Part model, mm, in its own coordinate system. A direction names the side the tool comes from. Give positions to 0.01 mm unless a question says otherwise; leave off trailing zeros. Order: outer loops, then holes, each group sorted by start corner. A loop starts at its lowest first (then second) coordinate and runs counter-clockwise, first axis right, second up. Notation, with made-up numbers: M 2,-29.5 L 16,-29.5 A20 ccw 16,3.5 Z; hole C -26,17 d9. An arc over 180 degrees is marked long. Return JSON: item names as keys, results as strings.
Autodesk Inventor part; units mm, degrees
ref_plane "YZ Plane" through (0, 0, 0) normal (1, 0, 0) x (0, 1, 0)
ref_plane "XZ Plane" through (0, 0, 0) normal (0, 1, 0) x (-1, 0, 0)
ref_plane "XY Plane" through (0, 0, 0) normal (0, 0, 1) x (1, 0, 0)
sketch "Boceto1" plane through (0, 0, 0) normal (0, 0, 1) x (1, 0, 0)
  line L0 (0, 0) -> (177, 0)
  line L1 (177, 0) -> (177, 127.5)
  line L2 (177, 127.5) -> (0, 127.5)
  line L3 (0, 127.5) -> (0, 0)
  line L4 (0, 127.5) -> (11.5, 127.5)
  line L5 (11.5, 127.5) -> (11.5, 116)
  line L6 (11.5, 116) -> (0, 116)
  line L7 (0, 116) -> (0, 127.5)
  line L8 (177, 0) -> (165.5, 0)
  line L9 (165.5, 0) -> (165.5, 11.5)
  line L10 (165.5, 11.5) -> (177, 11.5)
  line L11 (177, 11.5) -> (177, 0)
  line L12 (11.5, 116) -> (165.5, 116)
  line L13 (165.5, 116) -> (165.5, 11.5)
  line L14 (165.5, 11.5) -> (11.5, 11.5)
  line L15 (11.5, 11.5) -> (11.5, 116)
  dimension "d0" = 177
  dimension "d1" = 127.5
  dimension "d2" = 11.5
  dimension "d3" = 11.5
  dimension "d4" = 11.5
  dimension "d5" = 11.5
extrude "Extrusión1" add sketch "Boceto1" along normal blind 30 contours L3 L6 L15 L14 L9 L0 | L9 L10 L1 L0 | L3 L2 L5 L6 | L13 L12 L5 L2 L1 L10
sketch "Boceto2" plane through (0, 0, 30) normal (0, 0, 1) x (1, 0, 0)
  line L0 (11.5, 116) -> (6.5, 116)
  line L1 (6.5, 116) -> (6.5, 11.5)
  line L2 (6.5, 11.5) -> (11.5, 11.5)
  line L3 (11.5, 11.5) -> (11.5, 116)
  line L4 (165.5, 116) -> (170.5, 116)
  line L5 (170.5, 116) -> (170.5, 11.5)
  line L6 (170.5, 11.5) -> (165.5, 11.5)
  line L7 (165.5, 11.5) -> (165.5, 116)
  line L8 (11.5, 116) -> (165.5, 116)
  line L9 (165.5, 116) -> (165.5, 119.75)
  line L10 (165.5, 119.75) -> (11.5, 119.75)
  line L11 (11.5, 119.75) -> (11.5, 116)
  line L12 (11.5, 11.5) -> (165.5, 11.5)
  line L13 (165.5, 11.5) -> (165.5, 7.75)
  line L14 (165.5, 7.75) -> (11.5, 7.75)
  line L15 (11.5, 7.75) -> (11.5, 11.5)
  dimension "d30" = 5
  dimension "d31" = 5
  dimension "d32" = 104.5
  dimension "d33" = 3.75
  dimension "d34" = 3.75
extrude "Extrusión2" cut sketch "Boceto2" against normal blind 30 contours L3 L2 L1 L0 | L11 L10 L9 L8 | L12 L13 L14 L15 | L4 L5 L6 L7
sketch "Boceto3" plane through (0, 0, 30) normal (0, 0, 1) x (1, 0, 0)
  line L0 (177, 0) -> (171.25, 0)
  line L1 (171.25, 0) -> (171.25, 5.75)
  line L2 (171.25, 5.75) -> (177, 5.75)
  line L3 (177, 5.75) -> (177, 0)
  line L4 (0, 0) -> (5.75, 0)
  line L5 (5.75, 0) -> (5.75, 5.75)
  line L6 (5.75, 5.75) -> (0, 5.75)
  line L7 (0, 5.75) -> (0, 0)
  line L8 (0, 127.5) -> (5.75, 127.5)
  line L9 (5.75, 127.5) -> (5.75, 121.75)
  line L10 (5.75, 121.75) -> (0, 121.75)
  line L11 (0, 121.75) -> (0, 127.5)
  line L12 (177, 127.5) -> (171.25, 127.5)
  line L13 (171.25, 127.5) -> (171.25, 121.75)
  line L14 (171.25, 121.75) -> (177, 121.75)
  line L15 (177, 121.75) -> (177, 127.5)
  circle A0 centre (5.75, 121.75) radius 2
  circle A1 centre (171.25, 121.75) radius 2
  circle A2 centre (171.25, 5.75) radius 2
  circle A3 centre (5.75, 5.75) radius 2
  dimension "d16" = 5.75
  dimension "d17" = 5.75
  dimension "d18" = 5.75
  dimension "d19" = 5.75
  dimension "d20" = 5.75
  dimension "d21" = 5.75
  dimension "d22" = 5.75
  dimension "d23" = 5.75
  dimension "d24" = 4
  dimension "d25" = 4
  dimension "d26" = 4
  dimension "d27" = 4
extrude "Extrusión3" cut sketch "Boceto3" against normal blind 30 contours A2 L2 L1 | L1 L2 A2 | A3 L6 L5 | L5 L6 A3 | A0 L10 L9 | L9 L10 A0 | A1 L14 L13 | L13 L14 A1
sketch "Boceto4" plane through (0, 0, 0) normal (0, -1, 0) x (1, 0, 0)
  line L0 (0, 30) -> (21.5, 30)
  line L1 (21.5, 30) -> (21.5, 0)
  line L2 (21.5, 0) -> (0, 0)
  line L3 (0, 0) -> (0, 30)
  line L4 (0, 30) -> (177, 30)
  line L5 (177, 0) -> (155.5, 0)
  line L6 (155.5, 0) -> (155.5, 30)
  line L7 (155.5, 30) -> (177, 30)
  line L8 (177, 30) -> (177, 0)
  line L9 (0, 30) -> (21.5, 30)
  line L10 (21.5, 30) -> (21.5, 25)
  line L11 (21.5, 25) -> (0, 25)
  line L12 (0, 25) -> (0, 30)
  line L13 (0, 0) -> (21.5, 0)
  line L14 (21.5, 0) -> (21.5, 5)
  line L15 (21.5, 5) -> (0, 5)
  line L16 (0, 5) -> (0, 0)
  line L17 (0, 25) -> (21.5, 25)
  line L18 (21.5, 25) -> (21.5, 5)
  line L19 (21.5, 5) -> (0, 5)
  line L20 (0, 5) -> (0, 25)
  dimension "d35" = 21.5
  dimension "d36" = 21.5
  dimension "d37" = 5
  dimension "d38" = 5
extrude "Extrusión4" cut sketch "Boceto4" against normal blind 10.5 contours L11 L1 L15 L3
ref_plane "Plano de trabajo1" through (88.5, 0, 0) normal (-1, 0, 0) x (0, 0, 1)
ref_plane "Plano de trabajo2" through (11.5, 63.75, 30) normal (0, -1, 0) x (1, 0, 0)
mirror "Simetría1" about plane through (88.5, 0, 0) normal (-1, 0, 0) of "Extrusión4"
mirror "Simetría2" about plane through (11.5, 63.75, 30) normal (0, -1, 0) of "Extrusión4", "Simetría1"
sketch "Boceto5" plane through (0, 0, 0) normal (0, -1, 0) x (1, 0, 0)
  line L0 (21.5, 25) -> (155.5, 25)
  line L1 (155.5, 25) -> (155.5, 5)
  line L2 (155.5, 5) -> (21.5, 5)
  line L3 (21.5, 5) -> (21.5, 25)
  line L4 (21.5, 25) -> (31.5, 25)
  line L5 (31.5, 25) -> (31.5, 5)
  line L6 (31.5, 5) -> (21.5, 5)
  line L7 (21.5, 5) -> (21.5, 25)
  line L8 (155.5, 5) -> (147.5, 5)
  line L9 (147.5, 5) -> (147.5, 25)
  line L10 (147.5, 25) -> (155.5, 25)
  line L11 (155.5, 25) -> (155.5, 5)
  line L12 (31.5, 25) -> (147.5, 25)
  line L13 (147.5, 25) -> (147.5, 5)
  line L14 (147.5, 5) -> (31.5, 5)
  line L15 (31.5, 5) -> (31.5, 25)
  point P0 (0, 0)
  dimension "d41" = 10
  dimension "d42" = 8
extrude "Extrusión5" cut sketch "Boceto5" against normal blind 11.5 contours L0 L9 L2 L5
sketch "Boceto6" plane through (177, 0, 0) normal (1, 0, 0) x (0, 0, -1)
  line L0 (-25, 10.5) -> (-5, 10.5)
  line L1 (-5, 10.5) -> (-5, 18.5)
  line L2 (-5, 18.5) -> (-25, 18.5)
  line L3 (-25, 18.5) -> (-25, 10.5)
  line L4 (-25, 117) -> (-5, 117)
  line L5 (-5, 117) -> (-5, 109)
  line L6 (-5, 109) -> (-25, 109)
  line L7 (-25, 109) -> (-25, 117)
  line L8 (-25, 109) -> (-5, 109)
  line L9 (-5, 109) -> (-5, 18.5)
  line L10 (-5, 18.5) -> (-25, 18.5)
  line L11 (-25, 18.5) -> (-25, 109)
  point P0 (0, 0)
  dimension "d45" = 20
  dimension "d46" = 8
  dimension "d47" = 20
  dimension "d48" = 8
extrude "Extrusión6" cut sketch "Boceto6" against normal blind 200 contours L11 L6 L9 L2
properties part number "transillum_diffusor_partD2_v1"
Q1. Band-saw the part on B-B (x = 112.5). Give the cut face in (y, z), then the cut area to 3 significant figures.
Established:
{"outline": "M 0,0 L 7.75,0 L 7.75,5 L 0,5 Z; M 0,25 L 7.75,25 L 7.75,30 L 0,30 Z; M 119.75,0 L 127.5,0 L 127.5,30 L 119.75,30 Z", "area": "310 mm²"}
Q2. Band-saw the part on C-C (x = 149.5). Give the cut face in (y, z).
Established:
{"outline": "M 0,0 L 7.75,0 L 7.75,30 L 0,30 Z; M 119.75,0 L 127.5,0 L 127.5,30 L 119.75,30 Z"}
Q3. Two-plate mould, pull along Y, no slides. Class faces 1 (the cylindrical face through (169.252, 5.838, 2.535)), 2 (the flat face through (82, 7, 30)), 3 (the flat face through (6, 117, 15)): +Y half, -Y half, draft (parallel to the pull), parting line (faces both ways), or undercut.
Established:
{"face 1": "undercut", "face 2": "draft", "face 3": "+Y half"}
Q4. Probe line 1 along X through (y, z) = (121.75, 26.6); line 2 along Y through (x, z) = (171.25, 27.3); line 3 along Y through (x, z) = (123, 26.25). List the from-to ranges inside material, lowest first.
Established:
{"line 1": "x = 0 to 3.75, 7.75 to 169.25, 173.25 to 177", "line 2": "y = 0 to 3.75, 7.75 to 119.75, 123.75 to 127.5", "line 3": "y = 0 to 7.75, 119.75 to 127.5"}
Q5. Band-saw the part on A-A (y = 121.75). Give the cut face in (x, z), then the cut area to 3 significant figures.
Established:
{"outline": "M 0,0 L 3.75,0 L 3.75,5 L 0,5 Z; M 0,25 L 3.75,25 L 3.75,30 L 0,30 Z; M 7.75,0 L 169.25,0 L 169.25,5 L 155.5,5 L 155.5,25 L 169.25,25 L 169.25,30 L 7.75,30 L 7.75,25 L 21.5,25 L 21.5,5 L 7.75,5 Z; M 173.25,0 L 177,0 L 177,5 L 173.25,5 Z; M 173.25,25 L 177,25 L 177,30 L 173.25,30 Z", "area": "4,370 mm²"}
Q6. 3-axis set-ups, long thin cutter, end or side, ignore diameter. For faces 4 (the flat face through (11.5, 11, 19)), 5 (the flat face through (21.5, 124, 15)), 6 (the flat face through (174, 18.5, 15)), 7 (the flat face through (171, 117, 15)): which of +Z, -Z, +X, -X, +Y, -Y reach the whole face in a straight line?
Established:
{"face 4": "+Z, -Z", "face 5": "-X, +Y, -Y", "face 6": "+X, -X", "face 7": "+X, -X, +Y"}
Q7. Band-saw the part on D-D (y = 32). Give the cut face in (x, z), then the cut area to 3 significant figures.
Established:
{"outline": "M 0,0 L 6.5,0 L 6.5,5 L 0,5 Z; M 0,25 L 6.5,25 L 6.5,30 L 0,30 Z; M 170.5,0 L 177,0 L 177,5 L 170.5,5 Z; M 170.5,25 L 177,25 L 177,30 L 170.5,30 Z", "area": "130 mm²"}
Q8. Pin check, flat tips, straight feed: pin 1 (2.5 mm diameter, centred on x = 8.5, z = 18.5, fed in from +Y); pin 2 (8 mm diameter, centred on x = 107, z = 14.5, fed in from -Y); pin 3 (6 mm diameter, centred on x = 4, z = 14, fed in from -Y). Stop position of each tip, or through.
Established:
{"pin 1": "stops at y = 117", "pin 2": "stops at y = 119.75", "pin 3": "stops at y = 10.5"}
